from build123d import *

# Parameters (mm, degrees)
SKETCH1_R               = 7.5
BOSS_EXTRUDE1_DEPTH     = 15
SKETCH2_R               = 7.5
BOSS_EXTRUDE2_DEPTH     = 50
SKETCH3_W               = 50
SKETCH3_H               = 40
BOSS_EXTRUDE3_DEPTH     = 65
CUT_EXTRUDE2_DEPTH      = 96.372952141
SKETCH9_R               = 4
SKETCH9_R_2             = 10.5
CUT_EXTRUDE3_DEPTH      = 104.107953137
ESQUISSE1_R             = 2
ENL_V_MAT_EXTRU_1_DEPTH = 10
BOSS_EXTRU_1_START      = 5
ESQUISSE3_W             = 65
ESQUISSE3_H             = 50
ESQUISSE3_R             = 4
ESQUISSE3_W_2           = 42
ESQUISSE3_H_2           = 42
ESQUISSE3_R_2           = 1.5
ESQUISSE3_R_3           = 11
BOSS_EXTRU_1_DEPTH      = 5
BOSS_EXTRU_2_START      = 20
ESQUISSE3_4_W           = 65
ESQUISSE3_4_H           = 50
ESQUISSE3_4_R           = 4
ESQUISSE3_4_W_2         = 42
ESQUISSE3_4_H_2         = 42
BOSS_EXTRU_2_DEPTH      = 20
ESQUISSE3_5_R           = 1.5
ENL_V_MAT_EXTRU_4_DEPTH = 20


with BuildPart() as part:
    # Sketch1 → Boss-Extrude1 (new body)
    with BuildSketch(Plane.XY):
        with BuildLine():
            Line((0, 0), (50, 0))
            Line((50, 0), (50, 50))
            ThreePointArc((50, 50), (40.582575695, 63.228756555), (25, 58.660254038))
            ThreePointArc((25, 58.660254038), (9.417424305, 63.228756555), (0, 50))
            Line((0, 50), (0, 0))
        make_face()
        with Locations((36, 50)):
            Circle(SKETCH1_R, mode=Mode.SUBTRACT)
        with Locations((14, 50)):
            Circle(SKETCH1_R, mode=Mode.SUBTRACT)
    extrude(amount=BOSS_EXTRUDE1_DEPTH)

    # Sketch2 → Boss-Extrude2 (add)
    with BuildSketch(Plane.XY.offset(15)):
        with BuildLine():
            Line((0, 50), (0, 0))
            Line((0, 0), (25, 0))
            Line((25, 0), (25, 50))
            ThreePointArc((25, 50), (12.5, 62.5), (0, 50))
        make_face()
        with Locations((14, 50)):
            Circle(SKETCH2_R, mode=Mode.SUBTRACT)
    extrude(amount=BOSS_EXTRUDE2_DEPTH)

    # Sketch3 → Boss-Extrude3 (add)
    with BuildSketch(Plane(origin=(0, 0, 0), x_dir=(-1, 0, 0), z_dir=(0, 0, -1))):
        with Locations((-25, 20)):
            Rectangle(SKETCH3_W, SKETCH3_H)
    extrude(amount=-BOSS_EXTRUDE3_DEPTH)

    # Sketch2_3 → Cut-Extrude2 (cut, through all)
    with BuildSketch(Plane.XY.offset(15)):
        with BuildLine():
            ThreePointArc((50, 50), (37.5, 62.5), (25, 50))
            ThreePointArc((25, 50), (12.5, 62.5), (0, 50))
            ThreePointArc((0, 50), (9.417424305, 63.228756555), (25, 58.660254038))
            ThreePointArc((25, 58.660254038), (40.582575695, 63.228756555), (50, 50))
        make_face()
    extrude(amount=-CUT_EXTRUDE2_DEPTH, mode=Mode.SUBTRACT)

    # Sketch9 → Cut-Extrude3 (cut, through all)
    with BuildSketch(Plane.ZY):
        with Locations((58, 13)):
            Circle(SKETCH9_R)
        with Locations((7, 13)):
            Circle(SKETCH9_R)
        with Locations((7, 31)):
            Circle(SKETCH9_R)
        with Locations((58, 31)):
            Circle(SKETCH9_R)
        with Locations((32.5, 24)):
            Circle(SKETCH9_R_2)
    extrude(amount=-CUT_EXTRUDE3_DEPTH, mode=Mode.SUBTRACT)

    # Esquisse1 → Enl_v. mat.-Extru.1 (cut)
    with BuildSketch(Plane(origin=(0, 40, 0), x_dir=(1, 0, 0), z_dir=(0, 1, 0))):
        with Locations(Location((46, -42, 0), (0, 0, 270))):
            Circle(ESQUISSE1_R)
        with Locations(Location((46, -62, 0), (0, 0, 270))):
            Circle(ESQUISSE1_R)
    extrude(amount=-ENL_V_MAT_EXTRU_1_DEPTH, mode=Mode.SUBTRACT)

    # Esquisse3 → Boss.-Extru.1 (add)
    # profile 1 of 6: a face of its own
    with BuildSketch(Plane.ZY.offset(BOSS_EXTRU_1_START)):
        with Locations((32.5, 25)):
            Rectangle(ESQUISSE3_W, ESQUISSE3_H)
        with Locations((7, 31)):
            Circle(ESQUISSE3_R, mode=Mode.SUBTRACT)
        with Locations((58, 13)):
            Circle(ESQUISSE3_R, mode=Mode.SUBTRACT)
        with Locations((7, 13)):
            Circle(ESQUISSE3_R, mode=Mode.SUBTRACT)
        with Locations((58, 31)):
            Circle(ESQUISSE3_R, mode=Mode.SUBTRACT)
        with Locations((32.5, 23)):
            Rectangle(ESQUISSE3_W_2, ESQUISSE3_H_2, mode=Mode.SUBTRACT)
    # profile 2 of 6: a face of its own
    with BuildSketch(Plane.ZY.offset(BOSS_EXTRU_1_START)):
        with Locations((58, 13)):
            Circle(ESQUISSE3_R)
    # profile 3 of 6: a face of its own
    with BuildSketch(Plane.ZY.offset(BOSS_EXTRU_1_START)):
        with Locations((58, 31)):
            Circle(ESQUISSE3_R)
    # profile 4 of 6: a face of its own
    with BuildSketch(Plane.ZY.offset(BOSS_EXTRU_1_START)):
        with Locations((7, 31)):
            Circle(ESQUISSE3_R)
    # profile 5 of 6: a face of its own
    with BuildSketch(Plane.ZY.offset(BOSS_EXTRU_1_START)):
        with Locations((7, 13)):
            Circle(ESQUISSE3_R)
    # profile 6 of 6: a face of its own
    with BuildSketch(Plane.ZY.offset(BOSS_EXTRU_1_START)):
        with Locations((32.5, 23)):
            Rectangle(ESQUISSE3_W_2, ESQUISSE3_H_2)
        with Locations((17, 7.5)):
            Circle(ESQUISSE3_R_2, mode=Mode.SUBTRACT)
        with Locations((48, 7.5)):
            Circle(ESQUISSE3_R_2, mode=Mode.SUBTRACT)
        with Locations((48, 38.5)):
            Circle(ESQUISSE3_R_2, mode=Mode.SUBTRACT)
        with Locations((17, 38.5)):
            Circle(ESQUISSE3_R_2, mode=Mode.SUBTRACT)
        with Locations((32.5, 24)):
            Circle(ESQUISSE3_R_3, mode=Mode.SUBTRACT)
    extrude(amount=-BOSS_EXTRU_1_DEPTH)

    # Esquisse3_4 → Boss.-Extru.2 (add)
    # profile 1 of 5: a face of its own
    with BuildSketch(Plane.ZY.offset(BOSS_EXTRU_2_START)):
        with Locations((32.5, 25)):
            Rectangle(ESQUISSE3_4_W, ESQUISSE3_4_H)
        with Locations((7, 31)):
            Circle(ESQUISSE3_4_R, mode=Mode.SUBTRACT)
        with Locations((58, 13)):
            Circle(ESQUISSE3_4_R, mode=Mode.SUBTRACT)
        with Locations((7, 13)):
            Circle(ESQUISSE3_4_R, mode=Mode.SUBTRACT)
        with Locations((58, 31)):
            Circle(ESQUISSE3_4_R, mode=Mode.SUBTRACT)
        with Locations((32.5, 23)):
            Rectangle(ESQUISSE3_4_W_2, ESQUISSE3_4_H_2, mode=Mode.SUBTRACT)
    # profile 2 of 5: a face of its own
    with BuildSketch(Plane.ZY.offset(BOSS_EXTRU_2_START)):
        with Locations((58, 31)):
            Circle(ESQUISSE3_4_R)
    # profile 3 of 5: a face of its own
    with BuildSketch(Plane.ZY.offset(BOSS_EXTRU_2_START)):
        with Locations((58, 13)):
            Circle(ESQUISSE3_4_R)
    # profile 4 of 5: a face of its own
    with BuildSketch(Plane.ZY.offset(BOSS_EXTRU_2_START)):
        with Locations((7, 31)):
            Circle(ESQUISSE3_4_R)
    # profile 5 of 5: a face of its own
    with BuildSketch(Plane.ZY.offset(BOSS_EXTRU_2_START)):
        with Locations((7, 13)):
            Circle(ESQUISSE3_4_R)
    extrude(amount=-BOSS_EXTRU_2_DEPTH)

    # Esquisse3_5 → Enl_v. mat.-Extru.4 (cut)
    with BuildSketch(Plane.ZY):
        with Locations((17, 38.5)):
            Circle(ESQUISSE3_5_R)
        with Locations((48, 38.5)):
            Circle(ESQUISSE3_5_R)
        with Locations((48, 7.5)):
            Circle(ESQUISSE3_5_R)
        with Locations((17, 7.5)):
            Circle(ESQUISSE3_5_R)
    extrude(amount=-ENL_V_MAT_EXTRU_4_DEPTH, mode=Mode.SUBTRACT)


solid = part.part
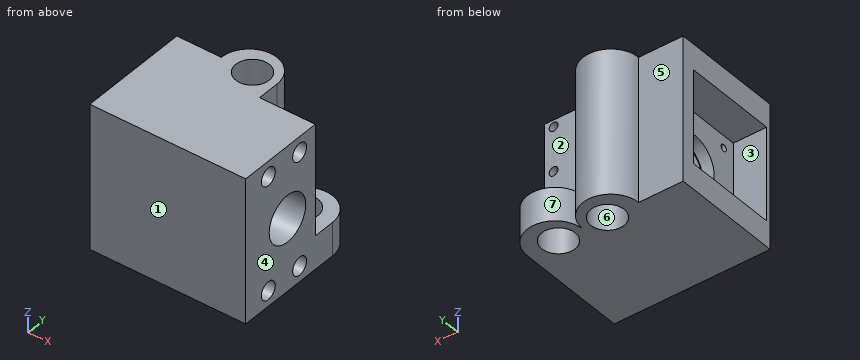
Verification items for the finished model (mm, model axes). Face numbers are marked on the shaded views. A direction names the side the tool comes from. Coordinates: 2 decimals unless noted, no trailing zeros. Order: outer loops, then holes, each group sorted by start corner. A loop starts at its lowest first (then second) coordinate and runs counter-clockwise, first axis right, second up.
1. Sectioned sample at D-D, the plane y = 16. Record the cut outline in (x, z), and give its area (3 significant figures).
Results found:
outline: (-20, 0) - (50, 0) - (50, 4.35) - (0, 4.35) - (0, 9.65) - (50, 9.65) - (50, 25.7) - (0, 25.7) - (0, 24.95) - (-5, 24.95) - (-5, 11.5) - (-20, 11.5) - close; (-20, 53.5) - (-5, 53.5) - (-5, 40.05) - (0, 40.05) - (0, 39.3) - (50, 39.3) - (50, 55.35) - (0, 55.35) - (0, 60.65) - (50, 60.65) - (50, 65) - (-20, 65) - close
area: 2,640 mm2
2. Sectioned sample at C-C, the plane x = 36. Record the cut outline in (y, z).
Results found:
outline: (0, 0) - (42.5, 0) - (42.5, 15) - (40, 15) - (40, 65) - (0, 65) - close; (57.5, 0) - (62.41, 0) - (62.41, 15) - (57.5, 15) - close; hole circle Ø8 at (13, 7); hole circle Ø8 at (13, 58); hole circle Ø21 at (24, 32.5); hole circle Ø8 at (31, 7); hole circle Ø8 at (31, 58)
3. Sectioned sample at A-A, the plane z = 32.5. Record the cut outline in (x, y).
Results found:
outline: (-20, 0) - (50, 0) - (50, 13.5) - (0, 13.5) - (0, 13) - (-5, 13) - (-5, 2) - (-20, 2) - close; (-20, 44) - (-5, 44) - (-5, 35) - (0, 35) - (0, 34.5) - (50, 34.5) - (50, 40) - (25, 40) - (25, 50) arc R12.5 ccw to (0, 50) - (-20, 50) - close; hole circle Ø15 at (14, 50)
4. Scan lines: line 1 (Y direction, x = 38.5, z = 58); line 2 (Y direction, x = 17.5, z = 6.5); line 3 (Z direction, x = 46, y = 33). Record each from-to range of solid material in increasing order.
Results found:
line 1: y = 0 to 9, 17 to 27, 35 to 40
line 2: y = 0 to 9.03, 16.97 to 27.03, 34.97 to 43.37, 56.63 to 61.46
line 3: z = 0 to 3.54, 10.46 to 27.09, 37.91 to 40, 44 to 54.54, 64 to 65
5. Sectioned sample at B-B, the plane x = 12.5. Give the number of separate pieces and of enclosed holes in the cut face, and give its area (3 significant figures).
Results found:
separate pieces: 2
enclosed holes: 9
area: 2,530 mm2
6. Set-up check for the marked faces 1, 2 and 3: record each of +Z, -Z, +X, -X, +Y, -Y from which the full face is reachable in a straight line by a thin tool's end or side.
Results found:
face 1: +Z, -Z, +X, -X, -Y
face 2: +Z, +X, +Y
face 3: -X
7. Go/stop test with flat-tipped pins: pin 1 Ø24 at (y, z) = (24, 32.5) entering from -X; pin 2 Ø9 at (y, z) = (13, 58) entering from +X; pin 3 Ø4 at (y, z) = (11.5, 57.5) entering from +X; pin 4 Ø1.5 at (x, z) = (13.5, 53) entering from +Y. Record where each tip stops, or that it passes through.
Results found:
pin 1: stops at x = -5
pin 2: stops at x = 50
pin 3: stops at x = 0
pin 4: stops at y = 62.5
8. Release check for a two-part mould opening along X. For the marked faces 4, 5, 6 and 7 record: +X half, -X half, draft (parallel to the pull), parting line (faces both ways), or undercut.
Results found:
face 4: +X half
face 5: draft
face 6: undercut
face 7: undercut
